Autodesk Inventor part; units mm, degrees
ref_plane "YZ Plane" through (0, 0, 0) normal (1, 0, 0) x (0, 1, 0)
ref_plane "XZ Plane" through (0, 0, 0) normal (0, 1, 0) x (-1, 0, 0)
ref_plane "XY Plane" through (0, 0, 0) normal (0, 0, 1) x (1, 0, 0)
sketch "Эскиз1" plane through (0, 0, 0) normal (0, 0, 1) x (1, 0, 0)
  circle A0 centre (0, 0) radius 2.5
  circle A1 centre (0, 0) radius 8
  dimension "d0" = 5
  dimension "d1" = 16
extrude "Выдавливание1" add sketch "Эскиз1" against normal blind 5
sketch "Эскиз4" plane through (0, 0, 0) normal (0, 0, 1) x (1, 0, 0)
  circle A0 centre (0, 0) radius 3
  circle A1 centre (0, 0) radius 7.5
  dimension "d8" = 6
  dimension "d9" = 15
extrude "Выдавливание2" cut sketch "Эскиз4" against normal blind 0.1
sketch "Эскиз5" plane through (0, 0, -5) normal (0, 0, -1) x (-1, 0, 0)
  circle A0 centre (0, 0) radius 3
  circle A1 centre (0, 0) radius 7.5
  dimension "d12" = 6
  dimension "d13" = 15
extrude "Выдавливание3" cut sketch "Эскиз5" against normal blind 0.1
sketch "Эскиз6" plane through (0, 0, -0.1) normal (0, 0, 1) x (1, 0, 0)
  point P0 (0, 0)
properties part number "625RS"
The listing builds one solid part. Answer for the finished solid, in the listing's coordinates (mm). A direction names the side the tool comes from. Give positions to 0.01 mm unless a question says otherwise; leave off trailing zeros. Order: outer loops, then holes, each group sorted by start corner. A loop starts at its lowest first (then second) coordinate and runs counter-clockwise, first axis right, second up. Notation, with made-up numbers: (64.5, -23.75) - (72.5, -23.75) arc R23 cw to (72.5, 9.25) - close; hole circle Ø5 at (41, 69). An arc over 180 degrees is marked (long way). Answer as CSV lines item,"result".
Q1. A cutting plane is placed at C-C, the plane z = -1.05. Determine the outline of the cut face in (x, y).
Answer key:
outline,"circle Ø16 at (0, 0); hole circle Ø5 at (0, 0)"
Q2. Which of the six approach directions +Z, -Z, +X, -X, +Y, -Y give full straight-line access (tool end or side, diameter ignored) to faces 4 (the face through (-0.1, -3.2, -0.1)), 5 (the face through (5, -6, 0))?
Answer key:
face 4,"+Z"
face 5,"+Z, +X, -X, +Y, -Y"
Q3. Straight lines are drawn through the part: L1, parallel to Y at x = 0, z = -4.85; L2, parallel to Y at x = 0, z = -4.95; L3, parallel to Z at x = 6, y = 1. For each, find the intervals that lie inside material, in ascending order.
Answer key:
L1,"y = -8 to -2.5, 2.5 to 8"
L2,"y = -8 to -7.5, -3 to -2.5, 2.5 to 3, 7.5 to 8"
L3,"z = -4.9 to -0.1"
Q4. Determine the mould class of faces 1 (the face through (5, -6, -5)), 2 (the face through (0.1, -3.2, -4.9)), 3 (the face through (-1.73, -7.81, -2.46)) for opening direction X: pulls with the +X half, pulls with the -X half, needs draft (parallel to the pull), parting line crosses it, or undercut.
Answer key:
face 1,"needs draft"
face 2,"undercut"
face 3,"parting line crosses it"
Q5. A cutting plane is placed at A-A, the plane y = 0. Determine the outline of the cut face in (x, z).
Answer key:
outline,"(-8, -5) - (-7.5, -5) - (-7.5, -4.9) - (-3, -4.9) - (-3, -5) - (-2.5, -5) - (-2.5, 0) - (-3, 0) - (-3, -0.1) - (-7.5, -0.1) - (-7.5, 0) - (-8, 0) - close; (2.5, -5) - (3, -5) - (3, -4.9) - (7.5, -4.9) - (7.5, -5) - (8, -5) - (8, 0) - (7.5, 0) - (7.5, -0.1) - (3, -0.1) - (3, 0) - (2.5, 0) - close"
Q6. Each of these flat-tipped pins is pushed along its axis until it touches: pin 1 Ø3 at (y, z) = (4, -2) entering from +X; pin 2 Ø2 at (x, z) = (-2, -1.5) entering from -Y. Where does it stop, or does it pass through?
Answer key:
pin 1,"stops at x = 7.6"
pin 2,"stops at y = -7.94"
Q7. A cutting plane is placed at D-D, the plane y = 5. Determine the outline of the cut face in (x, z) (3 decimals), and give its area (3 significant figures).
Answer key:
outline,"(-6.245, -5) - (-5.59, -5) - (-5.59, -4.9) - (5.59, -4.9) - (5.59, -5) - (6.245, -5) - (6.245, 0) - (5.59, 0) - (5.59, -0.1) - (-5.59, -0.1) - (-5.59, 0) - (-6.245, 0) - close"
area,"60.2 mm^2"
